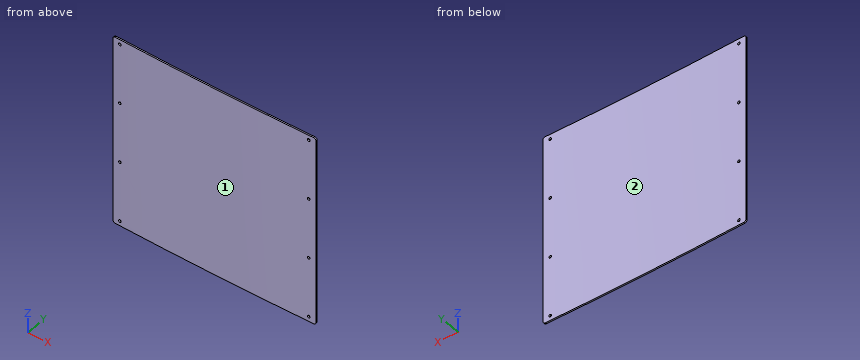
```python
from build123d import *

# Parameters (mm, degrees)
EXTRUS_O_FINA1_DEPTH  = 197.5
FILETE1_R             = 5
ESBO_O2_R             = 2.75
CORTE_EXTRUS_O1_DEPTH = 467.932004441
PADR_O_LINEAR2_COUNT  = 4
PADR_O_LINEAR2_PITCH  = 125


with BuildPart() as part:
    # Esboço1 → Extrusão-Fina1 (new, symmetric)
    with BuildSketch(Plane.XY):
        with BuildLine():
            ThreePointArc((0, 0), (211.5, -2.5), (423, 0))
            Line((423, 0), (423.070912078, -2.999161796))
            ThreePointArc((423.070912078, -2.999161796), (211.5, -5.5), (-0.070912078, -2.999161796))
            Line((-0.070912078, -2.999161796), (0, 0))
        make_face()
    extrude(amount=EXTRUS_O_FINA1_DEPTH, both=True)

    # Filete1
    filete1_edges = [part.edges().sort_by_distance(p)[0] for p in [
        (-0.035456039, -1.499580898, 197.5),
        (-0.035456039, -1.499580898, -197.5),
        (423.035456039, -1.499580898, -197.5),
        (423.035456039, -1.499580898, 197.5),
    ]]
    fillet(filete1_edges, radius=FILETE1_R)

    # Esboço2 → Corte-extrusão1 (cut, through all)
    with BuildSketch(Plane(origin=(0, 0, 0), x_dir=(1, 0, 0), z_dir=(0, 1, 0))):
        with Locations(Location((14.929087922, -187.5, 0), (0, 0, 270))):
            Circle(ESBO_O2_R)
        with Locations(Location((408, -187.5, 0), (0, 0, 270))):
            Circle(ESBO_O2_R)
    corte_extrus_o1 = extrude(amount=-CORTE_EXTRUS_O1_DEPTH, mode=Mode.SUBTRACT)

    # Padrão linear2: Corte-extrusão1 ×4
    with Locations(*[(0, 0, -i * PADR_O_LINEAR2_PITCH) for i in range(1, PADR_O_LINEAR2_COUNT)]):
        add(corte_extrus_o1, mode=Mode.SUBTRACT)


solid = part.part
```
The listing builds one solid part. Answer for the finished solid, in the listing's coordinates (mm). Face numbers are marked on the shaded views. A direction names the side the tool comes from. Coordinates: 2 decimals unless noted, no trailing zeros. Write each loop counter-clockwise with the first axis right and the second up, starting at its lowest first coordinate (ties: lowest second). Pieces come first, ordered by that corner, then holes.
Q1. Find the intervals of material crossed by line 1 along X through (y, z) = (-2.6, -187.5); line 2 along Z through (x, y) = (408, -2.3); line 3 along Y through (x, z) = (181.5, 24), in increasing order.
Returned:
line 1: x = -0.06 to 12.18, 17.68 to 405.25, 410.75 to 423.06
line 2: z = -197.5 to -190.25, -184.75 to -65.25, -59.75 to 59.75, 65.25 to 184.75, 190.25 to 197.5
line 3: y = -5.45 to -2.45
Q2. Which of the six approach directions +Z, -Z, +X, -X, +Y, -Y give full straight-line access (tool end or side, diameter ignored) to the marked faces 1 and 2?
Returned:
face 1: +Z, -Z, -Y
face 2: +Z, -Z, +Y
Q3. Section B-B, the plane x = 141 is taken. Write down the section's boundary in (y, z), then the cut area to 3 significant figures.
Returned:
outline: (-5.22, -197.5) - (-2.22, -197.5) - (-2.22, 197.5) - (-5.22, 197.5) - close
area: 1,190 mm2
Q4. Given P1, Ø9, axis at x = 14.93, z = -62.5, coming from the +Y side; P2, Ø1, axis at x = 161.5, z = 146.5, coming from the +Y side; P3, Ø7, axis at x = 408, z = -187.5, coming from the +Y side, each flat-ended and moving along its own axis, determine where each tip first touches the part or whether it passes through.
Returned:
P1: stops at y = -0.24
P2: stops at y = -2.36
P3: stops at y = -0.26
Q5. Section A-A, the plane z = -110.5 is taken. Write down the section's boundary in (x, y), then the cut area to 3 significant figures.
Returned:
outline: (-0.07, -3) arc R8950.7 ccw to (423.07, -3) - (423, 0) arc R8947.7 cw to (0, 0) - close
area: 1,270 mm2
